```python
from build123d import *

# Parameters (mm, degrees)
SKETCH1_R           = 4.5
BOSS_EXTRUDE1_DEPTH = 5
SKETCH2_W           = 20
SKETCH2_H           = 39
BOSS_EXTRUDE2_DEPTH = 25
CUT_EXTRUDE1_DEPTH  = 30
SKETCH4_R           = 2.5
SKETCH4_R_2         = 3
CUT_EXTRUDE2_DEPTH  = 30
FILLET1_R           = 5
FILLET2_R           = 1


with BuildPart() as part:
    # Sketch1 → Boss-Extrude1 (new body)
    with BuildSketch(Plane.XY):
        Polygon((-10, 10), (-10, -10), (10, -10), (10, 10), (10, 49), (-10, 49), align=None)
        Circle(SKETCH1_R, mode=Mode.SUBTRACT)
    extrude(amount=BOSS_EXTRUDE1_DEPTH)

    # Sketch2 → Boss-Extrude2 (add)
    with BuildSketch(Plane(origin=(0, 0, 0), x_dir=(-1, 0, 0), z_dir=(0, 0, -1))):
        with Locations((0, 29.5)):
            Rectangle(SKETCH2_W, SKETCH2_H)
    extrude(amount=BOSS_EXTRUDE2_DEPTH)

    # Sketch3 → Cut-Extrude1 (cut)
    with BuildSketch(Plane(origin=(10, 0, 0), x_dir=(0, 0, -1), z_dir=(1, 0, 0))):
        Polygon((0, 15), (-5, 15), (-5, 49), (20, 49), (20, 15), align=None)
    extrude(amount=-CUT_EXTRUDE1_DEPTH, mode=Mode.SUBTRACT)

    # Sketch4 → Cut-Extrude2 (cut)
    with BuildSketch(Plane.XY.offset(-20)):
        with Locations((0, 45)):
            Circle(SKETCH4_R)
        with Locations((0, 30)):
            Circle(SKETCH4_R_2)
    extrude(amount=-CUT_EXTRUDE2_DEPTH, mode=Mode.SUBTRACT)

    # Fillet1
    fillet1_edges = [part.edges().sort_by_distance(p)[0] for p in [
        (0, 15, -20),
    ]]
    fillet(fillet1_edges, radius=FILLET1_R)

    # Fillet2
    fillet2_edges = [part.edges().sort_by_distance(p)[0] for p in [
        (-10, 49, -22.5),
        (10, 49, -22.5),
        (0, 15, 5),
    ]]
    fillet(fillet2_edges, radius=FILLET2_R)


solid = part.part
```
Verification items for the finished model (mm, model axes). A direction names the side the tool comes from. Round coordinates to 2 decimals unless told otherwise and drop trailing zeros. Loops run counter-clockwise (first coordinate to the right, second up) from the corner with the lowest first, then second, coordinate; pieces in that order, holes last. Notation, with made-up numbers: (49, 10.25) -> (80, 10.25) arc R34 ccw to (80, 40.25) -> close; hole circle Ø3 at (27.5, 51). An arc over 180 degrees is marked (long way). Answer as a JSON object with one key per item and string values.
Q1. Section check B-B (z = -22). Record the boundary of the cut face in (x, y).
Data:
{"outline": "(-10, 10) -> (10, 10) -> (10, 48) arc R1 ccw to (9, 49) -> (-9, 49) arc R1 ccw to (-10, 48) -> close; hole circle Ø6 at (0, 30); hole circle Ø5 at (0, 45)"}
Q2. Go/stop test with flat-tipped pins: P1, Ø6, axis at x = 5, z = -14.5, coming from the -Y side; P2, Ø7, axis at x = 0, y = 0, coming from the -Z side; P3, Ø1.5, axis at x = 2, y = 18.5, coming from the +Z side; P4, Ø2, axis at x = 5, y = 8.5, coming from the -Z side. Record where each tip stops, or that it passes through.
Data:
{"P1": "stops at y = 10", "P2": "passes through", "P3": "stops at z = -19.47", "P4": "stops at z = 0"}
Q3. Section check C-C (x = 0). Record the boundary of the cut face in (y, z).
Data:
{"outline": "(-10, 0) -> (-4.5, 0) -> (-4.5, 5) -> (-10, 5) -> close; (4.5, 0) -> (10, 0) -> (10, -25) -> (27, -25) -> (27, -20) -> (20, -20) arc R5 cw to (15, -15) -> (15, 4) arc R1 ccw to (14, 5) -> (4.5, 5) -> close; (33, -25) -> (42.5, -25) -> (42.5, -20) -> (33, -20) -> close; (47.5, -25) -> (49, -25) -> (49, -20) -> (47.5, -20) -> close"}
Q4. Scan lines: line 1 (Y direction, x = 0, z = -22.45); line 2 (Z direction, x = -8.5, y = 36); line 3 (Y direction, x = -5.5, z = -0.25). Record each from-to range of solid material in increasing order. Write a range as from..to.
Data:
{"line 1": "y = 10..27, 33..42.5, 47.5..49", "line 2": "z = -25..-20", "line 3": "y = 10..15"}
Q5. Draft check along Y on faces 1 (the flat face through (0, 5, 5)), 2 (the flat face through (0, 10, -12)), 3 (the cylindrical face through (-2.21, 32.03, -22.46)). Enter one of: pulls with the +Y half, pulls with the -Y half, needs draft (parallel to the pull), parting line crosses it, or undercut.
Data:
{"face 1": "needs draft", "face 2": "pulls with the -Y half", "face 3": "undercut"}
Q6. Section check A-A (y = 30). Record the boundary of the cut face in (x, z).
Data:
{"outline": "(-10, -25) -> (-3, -25) -> (-3, -20) -> (-10, -20) -> close; (3, -25) -> (10, -25) -> (10, -20) -> (3, -20) -> close"}
Q7. Access from +Z, -Z, +X, -X, +Y, -Y to the whole of each face (thin tool, end or side, straight path). Record for faces 4 (the flat face through (-10, 14.6, -11)), 5 (the flat face through (0, 5, 0)), 6 (the flat face through (0, 35, -20)).
Data:
{"face 4": "+Z, -Z, -X, +Y, -Y", "face 5": "-Z, +X, -X, -Y", "face 6": "+Z, +X, -X, +Y"}
Q8. Section check D-D (x = -8). Record the boundary of the cut face in (y, z).
Data:
{"outline": "(-10, 0) -> (10, 0) -> (10, -25) -> (49, -25) -> (49, -20) -> (20, -20) arc R5 cw to (15, -15) -> (15, 4) arc R1 ccw to (14, 5) -> (-10, 5) -> close"}
